Read the model definition and answer for the solid it produces. Units are mm, in the model's axes. A direction names the side the tool comes from. Round coordinates to 2 decimals unless told otherwise and drop trailing zeros. Order: outer loops, then holes, each group sorted by start corner. A loop starts at its lowest first (then second) coordinate and runs counter-clockwise, first axis right, second up. Notation, with made-up numbers: (-35.5, -39.5) -> (11.5, -39.5) arc R15 cw to (11.5, -25.5) -> close; hole circle Ø7 at (48.5, 70.5). An arc over 180 degrees is marked (long way). One line per item, written item: value. Start each with the question number.
1. Flat-ended cylindrical pins translate along their axes: pin 1 Ø10 at (y, z) = (-1, 8.5) entering from -X; pin 2 Ø8 at (y, z) = (-11, 8) entering from -X; pin 3 Ø5 at (y, z) = (-0.5, 25.5) entering from -X. Find the tip coordinate at first contact, or state that the pin passes through.
2. For faces 5 (the face through (0, -5, -1.975)), 6 (the face through (-6, -15, 0)), 7 (the face through (28, 0, -14)), determine the directions among +Z, -Z, +X, -X, +Y, -Y from which every point of the face is accessible in a straight line to the end or side of a thin tool.
3. Section A-A (x = -30) is taken. Give the vertices of the cut face in (y, z).
4. The mould has two halves that part along X. Classify faces 1 (the face through (-9.9, -4.9, 9.9)), 2 (the face through (-0.086, -5.14, 2.473)), 3 (the face through (1, 5, 8)), 4 (the face through (18.707, -7.395, 24.719)): released by +X, released by -X, zero draft, split by the parting line, or undercut.
5. Section B-B (z = 0) is taken. State how many separate pieces and enclosed holes the cut face has, then the cut area to 3 significant figures.
6. Consider line 1 (Z direction, x = 7, y = -3.5); line 2 (Z direction, x = 1, y = -3.5) (3 decimals); line 3 (Z direction, x = 0, y = -1) (3 decimals). Determine where each line is inside the solid, lowest interval first.
from build123d import *

# Parameters (mm, degrees)
SKETCH1_R           = 37.5
BOSS_EXTRUDE1_DEPTH = 5
SKETCH10_R          = 31
BOSS_EXTRUDE2_DEPTH = 15
CUT_EXTRUDE1_DEPTH  = 57.678920244
CUT_EXTRUDE2_DEPTH  = 57.678920244


with BuildPart() as part:
    # Sketch1 → Boss-Extrude1 (new body)
    with BuildSketch(Plane(origin=(0, 0, 0), x_dir=(1, 0, 0), z_dir=(0, 1, 0))):
        with Locations(Location((0, 0, 0), (0, 0, 270))):
            Circle(SKETCH1_R)
    extrude(amount=BOSS_EXTRUDE1_DEPTH)

    # Sketch10 → Boss-Extrude2 (add)
    with BuildSketch(Plane.XZ):
        with Locations(Location((0, 0, 0), (0, 0, 270))):
            Circle(SKETCH10_R)
    extrude(amount=BOSS_EXTRUDE2_DEPTH)

    # Sketch11 → Cut-Extrude1 (cut, through all)
    with BuildSketch(Plane.XZ.offset(15)):
        with BuildLine():
            Line((1.491643389, -1.975), (-1.491643389, -1.975))
            ThreePointArc((-1.491643389, -1.975), (0, 2.475), (1.491643389, -1.975))
        make_face()
    extrude(amount=-CUT_EXTRUDE1_DEPTH, mode=Mode.SUBTRACT)

    # Sketch12 → Cut-Extrude2 (cut, through all)
    with BuildSketch(Plane(origin=(0, 5, 0), x_dir=(1, 0, 0), z_dir=(0, 1, 0))):
        with BuildLine():
            Line((-12.522960402, -11.550987883), (-7.276029472, -8.24800199))
            add(Edge.make_bspline(
                [(-18.566317366, 18.087986584), (-16.574063082, 19.6861494), (-14.373261885, 20.959086767), (-9.79610982, 22.776270096), (-7.408671534, 23.325251613), (-2.682384051, 23.701949314), (-0.331512749, 23.530934674), (4.117390892, 22.54012868), (6.227320203, 21.718005169), (10.027759886, 19.551591543), (11.728984463, 18.201550208), (14.596266579, 15.14457286), (15.770893072, 13.428953103), (17.527571222, 9.826499131), (18.115264822, 7.92879983), (18.700426824, 4.149147995), (18.700079831, 2.255101797), (18.166772453, -1.34708247), (17.632310064, -3.067469712), (16.13399267, -6.184277521), (15.165044903, -7.59200202), (12.933009073, -9.988675008), (11.661654701, -10.986949869), (8.976160145, -12.519251352), (7.551287211, -13.059754313), (4.709672005, -13.681053825), (3.280670849, -13.764842942), (0.565855338, -13.522749206), (-0.732647761, -13.196039768), (-3.080034254, -12.219492133), (-4.140875366, -11.565006492), (-5.944027576, -10.043678404), (-6.69667503, -9.168330698), (-7.276029472, -8.24800199)],
                knots=[0, 0, 0, 0, 0.0625, 0.0625, 0.125, 0.125, 0.1875, 0.1875, 0.25, 0.25, 0.3125, 0.3125, 0.375, 0.375, 0.4375, 0.4375, 0.5, 0.5, 0.5625, 0.5625, 0.625, 0.625, 0.6875, 0.6875, 0.75, 0.75, 0.8125, 0.8125, 0.875, 0.875, 0.9375, 0.9375, 1, 1, 1, 1], degree=3))
            Line((-18.566317366, 18.087986584), (-22.445875943, 22.924206724))
            add(Edge.make_bspline(
                [(-22.445875943, 22.924206724), (-19.969825826, 24.910464833), (-17.237941121, 26.492521157), (-11.506970883, 28.767783903), (-8.520553945, 29.456293243), (-2.555690408, 29.931708754), (0.409277257, 29.717850527), (6.07214005, 28.456686238), (8.756936396, 27.412613765), (13.639010184, 24.629622306), (15.824727512, 22.897648426), (19.54476833, 18.931495095), (21.070095492, 16.707358252), (23.373848964, 11.983006302), (24.146644363, 9.49504246), (24.923059123, 4.480059499), (24.924920169, 1.966413332), (24.208227547, -2.874432658), (23.491955176, -5.18832883), (21.450084705, -9.435838641), (20.130617856, -11.357409493), (17.041692734, -14.674176771), (15.281683474, -16.059679472), (11.501399671, -18.216650696), (9.493060749, -18.981663836), (5.416503734, -19.872974834), (3.361647035, -19.996666952), (-0.616520536, -19.641913768), (-2.526245675, -19.164989771), (-6.049307758, -17.699343634), (-7.65007538, -16.716185155), (-10.430976704, -14.369925494), (-11.600495296, -13.016362199), (-12.522960402, -11.550987883)],
                knots=[0, 0, 0, 0, 0.0625, 0.0625, 0.125, 0.125, 0.1875, 0.1875, 0.25, 0.25, 0.3125, 0.3125, 0.375, 0.375, 0.4375, 0.4375, 0.5, 0.5, 0.5625, 0.5625, 0.625, 0.625, 0.6875, 0.6875, 0.75, 0.75, 0.8125, 0.8125, 0.875, 0.875, 0.9375, 0.9375, 1, 1, 1, 1], degree=3))
        make_face()
    extrude(amount=-CUT_EXTRUDE2_DEPTH, mode=Mode.SUBTRACT)


solid = part.part
Answer:
1. pin 1: x = -37.33
1. pin 2: x = -30.74
1. pin 3: x = -29.58
2. face 5: +Y, -Y
2. face 6: +Z, -Z, +X, -X, -Y
2. face 7: -Y
3. outline: (-15, -7.81) -> (0, -7.81) -> (0, -22.5) -> (5, -22.5) -> (5, 22.5) -> (0, 22.5) -> (0, 7.81) -> (-15, 7.81) -> close
4. face 1: undercut
4. face 2: undercut
4. face 3: zero draft
4. face 4: split by the parting line
5. separate pieces: 3
5. enclosed holes: 0
5. area: 1,080 mm^2
6. line 1: -30.2 to -27.98, -21.23 to 13.15, 19.52 to 30.2
6. line 2: -30.984 to -29.495, -23.216 to -1.975, 2.264 to 13.529, 19.782 to 30.984
6. line 3: -31 to -29.62, -23.374 to -1.975, 2.475 to 13.328, 19.648 to 31
